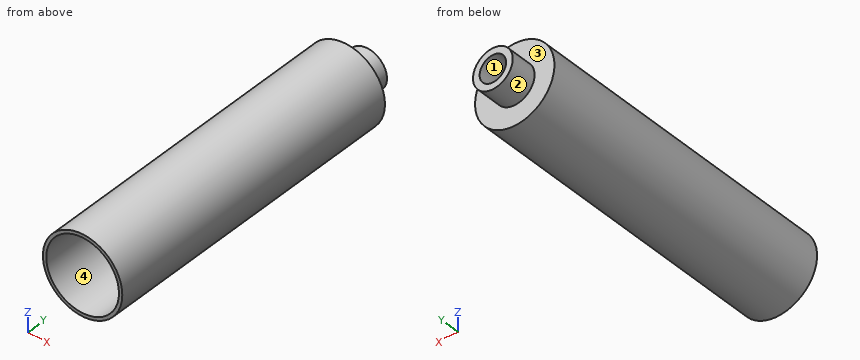
```python
from build123d import *

# Parameters (mm, degrees)
F0_R     = 38.1
F0_R_2   = 34.925
F1_DEPTH = 304.8
F2_DEPTH = 6.35
F3_R     = 19.05
F4_DEPTH = 25.4
F6_D     = 25.4
F6_DEPTH = 38.1


with BuildPart() as f1:
    # F0 (on Front) → F1 (new body)
    with BuildSketch(Plane.XZ):
        Circle(F0_R)
        Circle(F0_R_2, mode=Mode.SUBTRACT)
    extrude(amount=F1_DEPTH)

    # F0 (on Front) → F2 (join)
    with BuildSketch(Plane.XZ):
        Circle(F0_R_2)
    extrude(amount=F2_DEPTH)

    # F3 (on face) → F4 (join)
    with BuildSketch(Plane.XZ):
        Circle(F3_R)
    extrude(amount=-F4_DEPTH)

    # F6
    with Locations(Plane(origin=(0, 25.4, 0), x_dir=(-1, 0, 0), z_dir=(0, 1, 0))):
        with Locations((0, 0)):
            Hole(F6_D / 2, depth=F6_DEPTH)


solid = f1.part
```
Part model, mm, in its own coordinate system. Face numbers are marked on the shaded views. Round coordinates to 2 decimals unless told otherwise and drop trailing zeros. Write each loop counter-clockwise with the first axis right and the second up, starting at its lowest first coordinate (ties: lowest second). Pieces come first, ordered by that corner, then holes. Notation, with made-up numbers: (-29, 39) -> (2, 39) arc R21 ccw to (2, 71) -> close; hole circle Ø3 at (44, 29.5). An arc over 180 degrees is marked (long way). Return JSON: item names as keys, results as strings. Group by question number.
Q1. Saw through at B-B on x = 0. Write the cut outline in (y, z) (3 decimals), plus the area to 3 significant figures.
Q2. Saw through at D-D on x = 28. Write the cut outline in (y, z).
Q3. Saw through at A-A on z = 0. Write the cut outline in (x, y) (3 decimals), plus the area to 3 significant figures.
Q4. Saw through at C-C on y = -22. Write the cut outline in (x, z) (3 decimals).
Q5. Probe L1, parallel to Z at x = 0, y = -81 (3 decimals); L2, parallel to Z at x = 0, y = 11; L3, parallel to Y at x = 21, z = -2. List the from-to ranges inside material, lowest first. Write a range as [from, to].
Q6. Pin check, flat tips, straight feed: pin 1 (8 mm diameter, centred on x = -1, y = -256.5, fed in from -Z); pin 2 (1 mm diameter, centred on x = 26.5, y = -59, fed in from -Z); pin 3 (12 mm diameter, centred on y = -101, z = 9, fed in from -X). Stop position of each tip, or through.
Q7. Mould opens along Z. For the marked faces 1, 2, 3 and 4 say: pulls with the +Z half, pulls with the -Z half, needs draft (parallel to the pull), parting line crosses it, or undercut.
Answer:
{
 "1": {"outline": "(-304.8, -38.1) -> (0, -38.1) -> (0, -19.05) -> (25.4, -19.05) -> (25.4, -12.7) -> (-6.35, -12.7) -> (-6.35, -34.925) -> (-304.8, -34.925) -> close; (-304.8, 34.925) -> (-6.35, 34.925) -> (-6.35, 12.7) -> (25.4, 12.7) -> (25.4, 19.05) -> (0, 19.05) -> (0, 38.1) -> (-304.8, 38.1) -> close", "area": "2,540 mm2"},
 "2": {"outline": "(-304.8, -25.84) -> (0, -25.84) -> (0, 25.84) -> (-304.8, 25.84) -> (-304.8, 20.87) -> (-6.35, 20.87) -> (-6.35, -20.87) -> (-304.8, -20.87) -> close"},
 "3": {"outline": "(-38.1, -304.8) -> (-34.925, -304.8) -> (-34.925, -6.35) -> (-12.7, -6.35) -> (-12.7, 25.4) -> (-19.05, 25.4) -> (-19.05, 0) -> (-38.1, 0) -> close; (12.7, -6.35) -> (34.925, -6.35) -> (34.925, -304.8) -> (38.1, -304.8) -> (38.1, 0) -> (19.05, 0) -> (19.05, 25.4) -> (12.7, 25.4) -> close", "area": "2,540 mm2"},
 "4": {"outline": "circle Ø76.2 at (0, 0); hole circle Ø69.85 at (0, 0)"},
 "5": {"L1": "[-38.1, -34.925], [34.925, 38.1]", "L2": "[-19.05, -12.7], [12.7, 19.05]", "L3": "[-6.35, 0]"},
 "6": {"pin 1": "z = -38.1", "pin 2": "z = -27.85", "pin 3": "x = -37.98"},
 "7": {"face 1": "undercut", "face 2": "parting line crosses it", "face 3": "needs draft", "face 4": "undercut"}
}
